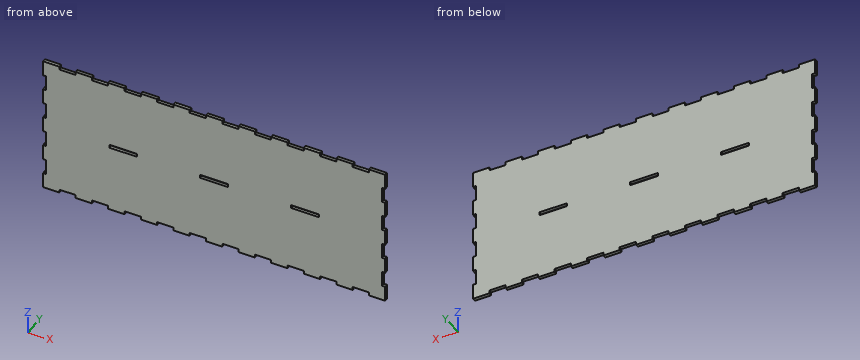
from build123d import *

# Parameters (mm, degrees)
F0_W     = 26
F0_H     = 3
F1_DEPTH = 3


with BuildPart() as f1:
    # F0 (on Front) → F1 (new body)
    with BuildSketch(Plane.XZ):
        Polygon((160, 61.999998), (160, 64.999998), (144.761429, 64.999998), (144.761429, 61.999998), (129.523333, 61.999998), (129.523333, 64.999998), (114.285238, 64.999998), (114.285238, 61.999998), (99.047143, 61.999998), (99.047143, 64.999998), (83.809048, 64.999998), (83.809048, 61.999998), (68.570952, 61.999998), (68.570952, 64.999998), (53.332952, 64.999998), (53.332952, 61.999998), (38.094952, 61.999998), (38.094952, 64.999998), (22.856952, 64.999998), (22.856952, 61.999998), (7.618857, 61.999998), (7.618857, 64.999998), (-7.619238, 64.999998), (-7.619238, 61.999998), (-22.857333, 61.999998), (-22.857333, 64.999998), (-38.095429, 64.999998), (-38.095429, 61.999998), (-53.333524, 61.999998), (-53.333524, 64.999998), (-68.571619, 64.999998), (-68.571619, 61.999998), (-83.809714, 61.999998), (-83.809714, 64.999998), (-99.047714, 64.999998), (-99.047714, 61.999998), (-114.285714, 61.999998), (-114.285714, 64.999998), (-129.52381, 64.999998), (-129.52381, 61.999998), (-144.761905, 61.999998), (-144.761905, 64.999998), (-160, 64.999998), (-160, 50.555558), (-157, 50.555558), (-157, 36.111118), (-160, 36.111118), (-160, 21.666678), (-157, 21.666678), (-157, 7.222238), (-160, 7.222238), (-160, 1.5), (-160, -1.5), (-160, -7.222202), (-157, -7.222202), (-157, -21.666642), (-160, -21.666642), (-160, -36.111082), (-157, -36.111082), (-157, -50.555526), (-160, -50.555526), (-160, -64.999998), (-144.761905, -64.999998), (-144.761905, -61.999998), (-129.52381, -61.999998), (-129.52381, -64.999998), (-114.285714, -64.999998), (-114.285714, -61.999998), (-99.047714, -61.999998), (-99.047714, -64.999998), (-83.809714, -64.999998), (-83.809714, -61.999998), (-68.571619, -61.999998), (-68.571619, -64.999998), (-53.333524, -64.999998), (-53.333524, -61.999998), (-38.095429, -61.999998), (-38.095429, -64.999998), (-22.857333, -64.999998), (-22.857333, -61.999998), (-7.619238, -61.999998), (-7.619238, -64.999998), (7.618857, -64.999998), (7.618857, -61.999998), (22.856952, -61.999998), (22.856952, -64.999998), (38.094952, -64.999998), (38.094952, -61.999998), (53.332952, -61.999998), (53.332952, -64.999998), (68.570952, -64.999998), (68.570952, -61.999998), (83.809048, -61.999998), (83.809048, -64.999998), (99.047143, -64.999998), (99.047143, -61.999998), (114.285238, -61.999998), (114.285238, -64.999998), (129.523333, -64.999998), (129.523333, -61.999998), (144.761429, -61.999998), (144.761429, -64.999998), (160, -64.999998), (160, -61.999998), (160, -50.555526), (157, -50.555526), (157, -36.111082), (160, -36.111082), (160, -21.666642), (157, -21.666642), (157, -7.222202), (160, -7.222202), (160, -1.5), (160, 1.5), (160, 7.222238), (157, 7.222238), (157, 21.666678), (160, 21.666678), (160, 36.111118), (157, 36.111118), (157, 50.555558), (160, 50.555558), align=None)
        with Locations((-85, 0)):
            Rectangle(F0_W, F0_H, mode=Mode.SUBTRACT)
        Rectangle(F0_W, F0_H, mode=Mode.SUBTRACT)
        with Locations((85, 0)):
            Rectangle(F0_W, F0_H, mode=Mode.SUBTRACT)
    extrude(amount=F1_DEPTH)


solid = f1.part
Geometry check sheet. Reference: the model listing, model coordinates, mm. Round coordinates to 2 decimals unless told otherwise and drop trailing zeros. Order: outer loops, then holes, each group sorted by start corner. A loop starts at its lowest first (then second) coordinate and runs counter-clockwise, first axis right, second up. Notation, with made-up numbers: M 55.25,54 L 114.25,54 A23 cw 114.25,76 Z; hole C -36,89.25 d10. An arc over 180 degrees is marked long. Write each question's results on one line, items separated by ' | '. Start each with the question number.
1. Cross-section at C-C on x = -43.5. Record the boundary of the cut face in (y, z).
2. Go/stop test with flat-tipped pins: P1, Ø0.9, axis at x = 46.5, y = -2, coming from the -Z side; P2, Ø1.5, axis at x = 104, y = -2, coming from the +Z side; P3, Ø1.5, axis at y = -1, z = 17, coming from the +X side. Record where each tip stops, or that it passes through.
3. Cross-section at D-D on z = 14.5. Record the boundary of the cut face in (x, y), plus the area to 3 significant figures.
4. Material ranges on L1, parallel to Z at x = 92, y = -1.2; L2, parallel to Z at x = -79, y = -1.95; L3, parallel to X at y = -1.2, z = 17, recorded low to high. Write a range as from..to.
5. Cross-section at A-A on x = -91.5. Record the boundary of the cut face in (y, z), plus the area to 3 significant figures.
6. Cross-section at B-B on y = -0.95. Give the number of separate pieces and of enclosed holes in the cut face, plus the area to 3 significant figures.
Resolved:
1) outline: M -3,-62 L 0,-62 L 0,62 L -3,62 Z
2) P1: z = -62 | P2: z = 62 | P3: x = 157
3) outline: M -157,-3 L 157,-3 L 157,0 L -157,0 Z | area: 942 mm2
4) L1: -65..-1.5, 1.5..65 | L2: -62..-1.5, 1.5..62 | L3: -157..157
5) outline: M -3,-65 L 0,-65 L 0,-1.5 L -3,-1.5 Z; M -3,1.5 L 0,1.5 L 0,65 L -3,65 Z | area: 381 mm2
6) separate pieces: 1 | enclosed holes: 3 | area: 40,100 mm2
